The model under review builds one solid part; all positions refer to its coordinate system, in mm. A direction names the side the tool comes from. Round coordinates to 2 decimals unless told otherwise and drop trailing zeros. Loops run counter-clockwise (first coordinate to the right, second up) from the corner with the lowest first, then second, coordinate; pieces in that order, holes last. Notation, with made-up numbers: (-1.5, 23) -> (56.5, 23) arc R12 ccw to (56.5, 46) -> close; hole circle Ø11 at (-25.5, -5.75). An arc over 180 degrees is marked (long way). Write each question's results on one line, items separated by ' | '. Start each with the question number.
Item 1: We need section A-A (x = 2.25). Give the boundary of the cut face in (y, z), and give its area (3 significant figures).
Item 2: For L1, parallel to Z at x = -10.75, y = 0.25; L2, parallel to Y at x = 9, z = 8.75; L3, parallel to X at y = -11.25, z = 6, list the stretches that pass through material, from the lowest coordinate up. Write a range as from..to.
Item 3: Tool access review of faces 1 (the cylindrical face through (12.686, 0.586, 4.893)), 2 (the cylindrical face through (11.81, 8.74, 4.44)): name each direction out of +Z, -Z, +X, -X, +Y, -Y from which nothing blocks a thin tool from reaching the whole face with its end or side.
Item 4: Mouldability with a two-part tool opening along Y and no side actions: class faces 3 (the cylindrical face through (0.49, -12.18, 4.89)), 4 (the cylindrical face through (3.682, 13.714, 4.437)), 5 (the flat face through (0, 0, 0)), 6 (the cylindrical face through (-3.682, -13.714, 4.437)) as pulls with the +Y half, pulls with the -Y half, needs draft (parallel to the pull), parting line crosses it, or undercut.
Item 5: We need section B-B (y = 11.5). Give the boundary of the cut face in (x, z), and give its area (3 significant figures).
Item 6: Clearance check with flat-ended pins moving along their axes: pin 1 Ø5 at (x, y) = (4.5, -4.5) entering from +Z; pin 2 Ø1 at (x, z) = (-2.5, 3.5) entering from -Y. State where each tip first meets the part, or that it passes through.
from build123d import *

# Parameters (mm, degrees)
F1_DEPTH = 0.9
F2_DEPTH = 9


with BuildPart() as f1:
    # F0 (on Top) → F1 (new body)
    with BuildSketch(Plane.XY):
        with BuildLine():
            ThreePointArc((0, 12.7), (-0.479927, 12.180703), (-0.999225, 12.66063))
            ThreePointArc((-0.999225, 12.66063), (-6.77809, 10.739995), (-10.998523, 6.35))
            ThreePointArc((-10.998523, 6.35), (-10.788762, 5.674722), (-11.464039, 5.464961))
            ThreePointArc((-11.464039, 5.464961), (-12.690154, -0.5), (-10.998523, -6.35))
            ThreePointArc((-10.998523, -6.35), (-10.308834, -6.505981), (-10.464815, -7.195669))
            ThreePointArc((-10.464815, -7.195669), (-5.912064, -11.239995), (0, -12.7))
            ThreePointArc((0, -12.7), (0.479927, -12.180703), (0.999225, -12.66063))
            ThreePointArc((0.999225, -12.66063), (6.77809, -10.739995), (10.998523, -6.35))
            ThreePointArc((10.998523, -6.35), (10.788762, -5.674722), (11.464039, -5.464961))
            ThreePointArc((11.464039, -5.464961), (12.690154, 0.5), (10.998523, 6.35))
            ThreePointArc((10.998523, 6.35), (10.308834, 6.505981), (10.464815, 7.195669))
            ThreePointArc((10.464815, 7.195669), (5.912064, 11.239995), (0, 12.7))
        make_face()
    extrude(amount=F1_DEPTH)

    # F0 (on Top) → F2 (join)
    with BuildSketch(Plane.XY):
        with BuildLine():
            ThreePointArc((0.99938, 14.164789), (0.517296, 14.682084), (0, 14.2))
            ThreePointArc((0, 14.2), (-2.670374, 13.946652), (-5.245461, 13.195648))
            ThreePointArc((-5.245461, 13.195648), (-5.90425, 13.452547), (-6.161149, 12.793758))
            ThreePointArc((-6.161149, 12.793758), (-8.457149, 11.406867), (-10.451375, 9.612948))
            ThreePointArc((-10.451375, 9.612948), (-11.156387, 9.558568), (-11.102007, 8.853555))
            ThreePointArc((-11.102007, 8.853555), (-12.568883, 6.607813), (-13.587265, 4.126285))
            ThreePointArc((-13.587265, 4.126285), (-14.198865, 3.771397), (-13.843976, 3.159797))
            ThreePointArc((-13.843976, 3.159797), (-14.191194, 0.5), (-14.032031, -2.177639))
            ThreePointArc((-14.032031, -2.177639), (-14.429083, -2.762745), (-13.843976, -3.159797))
            ThreePointArc((-13.843976, -3.159797), (-13.002766, -5.706844), (-11.697581, -8.050255))
            ThreePointArc((-11.697581, -8.050255), (-11.801444, -8.749692), (-11.102007, -8.853555))
            ThreePointArc((-11.102007, -8.853555), (-9.238981, -10.783378), (-7.046282, -12.328419))
            ThreePointArc((-7.046282, -12.328419), (-6.836385, -13.003655), (-6.161149, -12.793758))
            ThreePointArc((-6.161149, -12.793758), (-3.645302, -13.724131), (-0.99938, -14.164789))
            ThreePointArc((-0.99938, -14.164789), (-0.517296, -14.682084), (0, -14.2))
            ThreePointArc((0, -14.2), (2.670374, -13.946652), (5.245461, -13.195648))
            ThreePointArc((5.245461, -13.195648), (5.90425, -13.452547), (6.161149, -12.793758))
            ThreePointArc((6.161149, -12.793758), (8.457149, -11.406867), (10.451375, -9.612948))
            ThreePointArc((10.451375, -9.612948), (11.156387, -9.558568), (11.102007, -8.853555))
            ThreePointArc((11.102007, -8.853555), (12.568883, -6.607813), (13.587265, -4.126285))
            ThreePointArc((13.587265, -4.126285), (14.198865, -3.771397), (13.843976, -3.159797))
            ThreePointArc((13.843976, -3.159797), (14.191194, -0.5), (14.032031, 2.177639))
            ThreePointArc((14.032031, 2.177639), (14.429083, 2.762745), (13.843976, 3.159797))
            ThreePointArc((13.843976, 3.159797), (13.002766, 5.706844), (11.697581, 8.050255))
            ThreePointArc((11.697581, 8.050255), (11.801444, 8.749692), (11.102007, 8.853555))
            ThreePointArc((11.102007, 8.853555), (9.238981, 10.783378), (7.046282, 12.328419))
            ThreePointArc((7.046282, 12.328419), (6.836385, 13.003655), (6.161149, 12.793758))
            ThreePointArc((6.161149, 12.793758), (3.645302, 13.724131), (0.99938, 14.164789))
        make_face()
        with BuildLine():
            ThreePointArc((-10.998523, 6.35), (-6.77809, 10.739995), (-0.999225, 12.66063))
            ThreePointArc((-0.999225, 12.66063), (-0.479927, 12.180703), (0, 12.7))
            ThreePointArc((0, 12.7), (5.912064, 11.239995), (10.464815, 7.195669))
            ThreePointArc((10.464815, 7.195669), (10.308834, 6.505981), (10.998523, 6.35))
            ThreePointArc((10.998523, 6.35), (12.690154, 0.5), (11.464039, -5.464961))
            ThreePointArc((11.464039, -5.464961), (10.788762, -5.674722), (10.998523, -6.35))
            ThreePointArc((10.998523, -6.35), (6.77809, -10.739995), (0.999225, -12.66063))
            ThreePointArc((0.999225, -12.66063), (0.479927, -12.180703), (0, -12.7))
            ThreePointArc((0, -12.7), (-5.912064, -11.239995), (-10.464815, -7.195669))
            ThreePointArc((-10.464815, -7.195669), (-10.308834, -6.505981), (-10.998523, -6.35))
            ThreePointArc((-10.998523, -6.35), (-12.690154, -0.5), (-11.464039, 5.464961))
            ThreePointArc((-11.464039, 5.464961), (-10.788762, 5.674722), (-10.998523, 6.35))
        make_face(mode=Mode.SUBTRACT)
    extrude(amount=F2_DEPTH)


solid = f1.part
Here are the results:
1) outline: (-14.02, 0) -> (14.02, 0) -> (14.02, 9) -> (12.5, 9) -> (12.5, 0.9) -> (-12.5, 0.9) -> (-12.5, 9) -> (-14.02, 9) -> close | area: 49.9 mm2
2) L1: z = 0..0.9 | L2: y = -10.98..-8.96, 8.96..10.98 | L3: x = -8.66..-5.89, 5.89..8.66
3) face 1: +Z | face 2: +Z, -Z
4) face 3: undercut | face 4: pulls with the +Y half | face 5: needs draft | face 6: pulls with the -Y half
5) outline: (-8.33, 0) -> (8.33, 0) -> (8.33, 9) -> (5.39, 9) -> (5.39, 0.9) -> (-5.39, 0.9) -> (-5.39, 9) -> (-8.33, 9) -> close | area: 62.6 mm2
6) pin 1: stops at z = 0.9 | pin 2: stops at y = -14.06
